Model file for the job. Use its own axes, mm. A direction names the side the tool comes from. Round coordinates to 2 decimals unless told otherwise and drop trailing zeros. Order: outer loops, then holes, each group sorted by start corner. A loop starts at its lowest first (then second) coordinate and runs counter-clockwise, first axis right, second up. Notation, with made-up numbers: M 84.5,68.25 L 108.5,68.25 A11 ccw 108.5,83.25 Z; hole C -30.5,7 d2. An arc over 180 degrees is marked long. Return JSON: item names as keys, results as strings. Group by question number.
Item 1: Probe line 1 along Z through (x, y) = (19.65, 0); line 2 along Z through (x, y) = (16, 0); line 3 along X through (y, z) = (47, 4.25). List the from-to ranges inside material, lowest first.
Item 2: Slice it at A-A on z = 0. Give the number of separate pieces and of enclosed holes in the cut face, then the cut area to 3 significant figures.
Item 3: Pull direction Y, two halves, no side cores. Call faces 1 (the face through (16.4, 37.5, 0.2)), 2 (the face through (20, -4, 0)), 3 (the face through (16.28, -1.5, 0.07)): pulls with the +Y half, pulls with the -Y half, needs draft (parallel to the pull), parting line crosses it, or undercut.
Item 4: Slice it at B-B on y = 39. Write the cut outline in (x, z), then the cut area to 3 significant figures.
Item 5: Which spindle directions (+Z, -Z, +X, -X, +Y, -Y) get a long thin tool onto all of the face, cutting with end or side? Do faces 4 (the face through (18.5, 0, -2)), 5 (the face through (6, -1, -2)), 6 (the face through (1.5, 0, -2)), 7 (the face through (10, 50, 11)), 8 (the face through (6, 48, 0)). Say none if no direction does.
Item 6: Pin check, flat tips, straight feed: pin 1 Ø2 at (x, z) = (11, 9.5) entering from -Y; pin 2 Ø3.5 at (y, z) = (0, 0) entering from -X; pin 3 Ø5 at (y, z) = (13, 6.5) entering from +X; pin 4 Ø2.5 at (y, z) = (50, 0) entering from +X. Stop position of each tip, or through.
Item 7: Slice it at D-D on z = -5.5. Write the cut outline in (x, y).
Item 8: Slice it at C-C on x = 4.75. Write the cut outline in (y, z), then the cut area to 3 significant figures.
from build123d import *

# Parameters (mm, degrees)
F1_DEPTH  = 6
F3_DEPTH  = 8
F5_DEPTH  = 6
F6_R      = 12.5
F7_DEPTH  = 6
F8_R      = 12.5
F9_DEPTH  = 6
F11_DEPTH = 14.001
F12_R     = 1.5
F13_DEPTH = 20.001
F14_R     = 2.5
F15_DEPTH = 1.5
F16_R     = 2.5
F17_DEPTH = 1.5
F18_R     = 82.8644231172
F19_DEPTH = 12.5


with BuildPart() as f1:
    # F0 (on Right) → F1 (new body)
    with BuildSketch(Plane.YZ):
        with BuildLine():
            ThreePointArc((45.7146496628, 11.7424772722), (24.2728942701, 7.4219237759), (2.5168433046, 9.6780938092))
            ThreePointArc((2.5168433046, 9.6780938092), (-10, 0), (2.5168433046, -9.6780938092))
            ThreePointArc((2.5168433046, -9.6780938092), (24.2728942701, -7.4219237759), (45.7146496628, -11.7424772722))
            ThreePointArc((45.7146496628, -11.7424772722), (62.5, 0), (45.7146496628, 11.7424772722))
        make_face()
    extrude(amount=F1_DEPTH)

    # F2 (on face) → F3 (join)
    with BuildSketch(Plane.YZ.offset(6)):
        with BuildLine():
            ThreePointArc((45.7146496628, 11.7424772722), (24.2728942701, 7.4219237759), (2.5168433046, 9.6780938092))
            ThreePointArc((2.5168433046, 9.6780938092), (1.2686729105, 9.919196996), (0, 10))
            Line((0, 10), (0, 8))
            ThreePointArc((0, 8), (4.0630120127, 6.8914391374), (7, 3.8729833462))
            Line((7, 3.8729833462), (13.4120563723, -7.716117508))
            ThreePointArc((13.4120563723, -7.716117508), (29.7917342094, -7.8970456319), (45.7146496628, -11.7424772722))
            ThreePointArc((45.7146496628, -11.7424772722), (62.5, 0), (45.7146496628, 11.7424772722))
        make_face()
    extrude(amount=F3_DEPTH)

    # F4 (on face) → F5 (join)
    with BuildSketch(Plane.YZ.offset(14)):
        with BuildLine():
            ThreePointArc((2.5168433046, 9.6780938092), (1.2686729105, 9.919196996), (0, 10))
            ThreePointArc((0, 10), (-9.919196996, -1.2686729105), (2.5168433046, -9.6780938092))
            ThreePointArc((2.5168433046, -9.6780938092), (7.9270301673, -8.4893073841), (13.4120563723, -7.716117508))
            ThreePointArc((13.4120563723, -7.716117508), (29.7917342094, -7.8970456319), (45.7146496628, -11.7424772722))
            ThreePointArc((45.7146496628, -11.7424772722), (62.5, 0), (45.7146496628, 11.7424772722))
            ThreePointArc((45.7146496628, 11.7424772722), (24.2728942701, 7.4219237759), (2.5168433046, 9.6780938092))
        make_face()
    extrude(amount=F5_DEPTH)

    # F6 (on face) → F7 (cut)
    with BuildSketch(Plane.YZ.offset(20)):
        with Locations((50, 0)):
            Circle(F6_R)
    extrude(amount=-F7_DEPTH, mode=Mode.SUBTRACT)

    # F8 (on face) → F9 (cut)
    with BuildSketch(Plane(origin=(0, 0, 0), x_dir=(0, -1, 0), z_dir=(-1, 0, 0))):
        with Locations((-50, 0)):
            Circle(F8_R)
    extrude(amount=-F9_DEPTH, mode=Mode.SUBTRACT)

    # F10 (on face) → F11 (cut, through all)
    with BuildSketch(Plane.YZ.offset(14)):
        with BuildLine():
            Line((55, -7.4833147735), (47.7871856146, -12.3025790994))
            ThreePointArc((47.7871856146, -12.3025790994), (62.4505469507, -1.1108017956), (50, 12.5))
            Line((50, 12.5), (50, 9))
            ThreePointArc((50, 9), (58.6124860802, 2.6124860802), (55, -7.4833147735))
        make_face()
    extrude(amount=-F11_DEPTH, mode=Mode.SUBTRACT)

    # F12 (on face) → F13 (cut, through all)
    with BuildSketch(Plane.YZ.offset(20)):
        Circle(F12_R)
        with Locations((50, 0)):
            Circle(F12_R)
    extrude(amount=-F13_DEPTH, mode=Mode.SUBTRACT)

    # F14 (on face) → F15 (cut)
    with BuildSketch(Plane.YZ.offset(20)):
        Circle(F14_R)
    extrude(amount=-F15_DEPTH, mode=Mode.SUBTRACT)

    # F16 (on face) → F17 (cut)
    with BuildSketch(Plane(origin=(0, 0, 0), x_dir=(0, -1, 0), z_dir=(-1, 0, 0))):
        Circle(F16_R)
    extrude(amount=-F17_DEPTH, mode=Mode.SUBTRACT)

    # F18 (on Top) → F19 (cut, symmetric)
    with BuildSketch(Plane.XY):
        with Locations((-80, 24.1157464837)):
            Circle(F18_R)
        with Locations((100, 24.1157464837)):
            Circle(F18_R)
    extrude(amount=F19_DEPTH, both=True, mode=Mode.SUBTRACT)


solid = f1.part
Output values:
{
 "1": {"line 1": "-10 to -2.5, 2.5 to 10", "line 2": "-10 to -1.5, 1.5 to 10", "line 3": "6 to 14"},
 "2": {"separate pieces": "4", "enclosed holes": "0", "area": "753 mm²"},
 "3": {"face 1": "pulls with the +Y half", "face 2": "needs draft", "face 3": "undercut"},
 "4": {"outline": "M 1.52,-9.65 L 18.48,-9.65 L 18.48,-5.94 L 14,-5.94 L 14,5.94 L 18.48,5.94 L 18.48,9.65 L 1.52,9.65 L 1.52,5.94 L 6,5.94 L 6,-5.94 L 1.52,-5.94 Z", "area": "221 mm²"},
 "5": {"face 4": "+X", "face 5": "-Z, -Y", "face 6": "-X", "face 7": "+Z, +X, -X, +Y", "face 8": "-X, +Y"},
 "6": {"pin 1": "y = 0", "pin 2": "x = 1.5", "pin 3": "x = 18.26", "pin 4": "through"},
 "7": {"outline": "M 0,-8.35 L 6,-8.35 L 6,12.19 L 14,12.19 L 14,-8.35 L 20,-8.35 L 20,2.52 A82.86 cw 18.44,38.78 L 14,38.78 L 14,57.12 L 6,57.12 L 6,38.78 L 1.56,38.78 A82.86 cw 0,2.52 Z"},
 "8": {"outline": "M 2.52,-9.68 A72.66 cw 45.71,-11.74 A12.5 cw 45.71,11.74 A72.66 cw 2.52,9.68 A10 ccw long Z; hole C 0,0 d3", "area": "794 mm²"}
}
